from build123d import *

# Parameters (mm, degrees)
SKETCH1_W               = 8
SKETCH1_H               = 8
BOSS_EXTRUDE1_DEPTH     = 3
CUT_EXTRUDE1_DEPTH      = 12.704699911
CUT_EXTRUDE1_DEPTH_BACK = 12.704699911
CUT_EXTRUDE2_DEPTH      = 11
SKETCH4_R               = 1.75
CUT_EXTRUDE3_DEPTH      = 0.4
SKETCH5_W               = 8
SKETCH5_H               = 1
BOSS_EXTRUDE2_DEPTH     = 2
FILLET1_R               = 4
CUT_EXTRUDE4_DEPTH      = 0.4


with BuildPart() as part:
    # Sketch1 → Boss-Extrude1 (new body)
    with BuildSketch(Plane(origin=(0, 0, 0), x_dir=(1, 0, 0), z_dir=(0, 1, 0))):
        with Locations((4, 4)):
            Rectangle(SKETCH1_W, SKETCH1_H)
    extrude(amount=BOSS_EXTRUDE1_DEPTH)

    # Sketch2 → Cut-Extrude1 (cut, two sides: drawn at the far end of the back side and taken through both)
    with BuildSketch(Plane.XY.offset(-CUT_EXTRUDE1_DEPTH_BACK)):
        Polygon((0, 0), (0.6, 3), (0, 3), align=None)
        Polygon((8, 0), (7.4, 3), (8, 3), align=None)
    extrude(amount=CUT_EXTRUDE1_DEPTH + CUT_EXTRUDE1_DEPTH_BACK, mode=Mode.SUBTRACT)

    # Sketch3 → Cut-Extrude2 (cut)
    with BuildSketch(Plane(origin=(0, 0, 0), x_dir=(0, 0, -1), z_dir=(1, 0, 0))):
        Polygon((0, 0), (0.6, 3), (0, 3), align=None)
        Polygon((8, 3), (7.4, 3), (8, 0), align=None)
    extrude(amount=CUT_EXTRUDE2_DEPTH, mode=Mode.SUBTRACT)

    # Sketch4 → Cut-Extrude3 (cut)
    with BuildSketch(Plane.XZ):
        with Locations(Location((4, -3.75, 0), (0, 0, 270))):
            Circle(SKETCH4_R)
    extrude(amount=-CUT_EXTRUDE3_DEPTH, mode=Mode.SUBTRACT)

    # Sketch5 → Boss-Extrude2 (add)
    with BuildSketch(Plane.XZ):
        with Locations((4, -7.5)):
            Rectangle(SKETCH5_W, SKETCH5_H)
    extrude(amount=BOSS_EXTRUDE2_DEPTH)

    # Fillet1
    # the kernel refuses this fillet: 4 mm, written as the material it takes off along each edge
    with BuildSketch(Plane(origin=(8, -2, -16.660254038), x_dir=(0, 1, 0), z_dir=(0, 0, 1)), Plane(origin=(0, -2, 1.660254038), x_dir=(0, 1, 0), z_dir=(0, 0, -1))) as fillet1_piece_1:
        with BuildLine():
            CenterArc((4, 3.464101615), FILLET1_R, 180, 60)
            Line((0, 3.464101615), (-0.08, 3.464101615))
            Line((-0.08, 3.464101615), (-0.08, 0))
            Line((-0.08, 0), (0, -0.08))
            ThreePointArc((0, -0.08), (1, -0.08), (1.96, -0.069282032))
            Line((1.96, -0.069282032), (2, 0))
        make_face()
    extrude(amount=18.320508076, mode=Mode.SUBTRACT)

    # Sketch6 → Cut-Extrude4 (cut)
    with BuildSketch(Plane(origin=(0, 3, 0), x_dir=(1, 0, 0), z_dir=(0, 1, 0))):
        Polygon((3.605424489, 1.979723732), (2.126257822, 5.979723732), (2.938757822, 5.979723732), (3.998052694, 3.005364758), (5.053341155, 5.979723732), (5.869847566, 5.979723732), (4.396289873, 1.979723732), align=None)
    extrude(amount=-CUT_EXTRUDE4_DEPTH, mode=Mode.SUBTRACT)


solid = part.part
The model under review builds one solid part; all positions refer to its coordinate system, in mm. A direction names the side the tool comes from. Round coordinates to 2 decimals unless told otherwise and drop trailing zeros. Loops run counter-clockwise (first coordinate to the right, second up) from the corner with the lowest first, then second, coordinate; pieces in that order, holes last. Notation, with made-up numbers: M 60,37.25 L 85,37.25 A22 cw 85,71.25 Z; hole C 2.25,38.5 d1. An arc over 180 degrees is marked long. Answer as CSV lines item,"result". Start each with the question number.
Item 1: Consider section D-D (y = -1.1). Write out the cut boundary in (x, z).
Item 2: Wall thickness on line 1 (Y direction, x = 7, z = -6); line 2 (Z direction, x = 1.5, y = -0.5); line 3 (X direction, y = 0.2, z = -3.75): over which ranges is each line inside the solid? List them lowest first. Write a range as [from, to].
Item 3: Consider section C-C (x = 0.5). Write out the cut boundary in (y, z).
Item 4: Mouldability with a two-part tool opening along Z and no side actions: class faces 6 (the face through (2.876, 2.803, -3.952)), 7 (the face through (7.7, 1.5, -4.1)), 8 (the face through (4, -1, -7)), 9 (the face through (4.4, 2.6, -3.6)) as released by +Z, released by -Z, zero draft, split by the parting line, or undercut.
Item 5: Consider section A-A (x = 7.75). Write out the cut boundary in (y, z), then the cut area to 3 significant figures.
Item 6: For faces 1 (the face through (4, 0.4, -4)), 2 (the face through (3, 0, -2)), 3 (the face through (4, -1, -8)), 4 (the face through (4, -2, -7.5)), 5 (the face through (5.143, 2.803, -4.008)), list the 3-axis set-ups (+Z, -Z, +X, -X, +Y, -Y) from which the entire face can be reached by the end or side of a thin tool; tool diameter is ignored.
Item 7: Insertion check: P1, Ø3, axis at x = 4.5, y = 2, coming from the -Z side; P2, Ø1, axis at y = 2.5, z = -5.5, coming from the -X side; P3, Ø1, axis at x = 2, y = -1, coming from the +Z side. Each pin has a flat end and moves straight along its axis. Give the tip position at first contact, or say it passes through.
Item 8: Consider section B-B (z = -3.5). Write out the cut boundary in (x, y).
Answer:
1,outline,"M 0.94,-8 L 7.06,-8 L 7.06,-7 L 0.94,-7 Z"
2,line 1,"y = [0, 3]"
2,line 2,"z = [-8, -7]"
2,line 3,"x = [0.04, 2.25], [5.75, 7.96]"
3,outline,"M -0.69,-8 L 0,-8 L 2.5,-7.5 L 2.5,-0.5 L 0,0 L 0,-7 L -0.69,-7 Z"
4,face 6,"undercut"
4,face 7,"zero draft"
4,face 8,"released by +Z"
4,face 9,"undercut"
5,outline,"M -0.38,-8 L 0,-8 L 1.25,-7.75 L 1.25,-0.25 L 0,0 L 0,-7 L -0.38,-7 Z"
5,area,"10.1 mm^2"
6,face 1,"-Y"
6,face 2,"+Z, +X, -X, -Y"
6,face 3,"-Z, +X, -X, +Y, -Y"
6,face 4,"+Z, -Z, +X, -X, -Y"
6,face 5,"+Y"
7,P1,"stops at z = -7.9"
7,P2,"stops at x = 0.4"
7,P3,"stops at z = -7"
8,outline,"M 0,0 L 2.27,0 L 2.27,0.4 L 5.73,0.4 L 5.73,0 L 8,0 L 7.4,3 L 4.96,3 L 4.96,2.6 L 4.17,2.6 L 4.17,3 L 3.82,3 L 3.82,2.6 L 3.04,2.6 L 3.04,3 L 0.6,3 Z"
